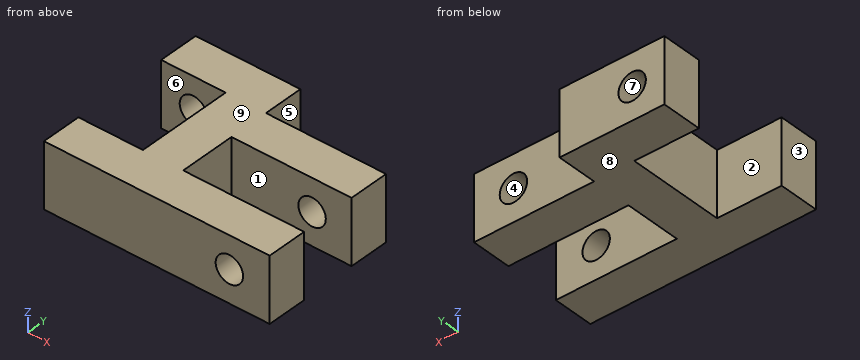
Autodesk Inventor part; units mm, degrees
ref_plane "YZ Plane" through (0, 0, 0) normal (1, 0, 0) x (0, 1, 0)
ref_plane "XZ Plane" through (0, 0, 0) normal (0, 1, 0) x (-1, 0, 0)
ref_plane "XY Plane" through (0, 0, 0) normal (0, 0, 1) x (1, 0, 0)
sketch "Sketch1" plane through (0, 0, 0) normal (0, 0, 1) x (1, 0, 0)
  line L0 (0, 0) -> (15, 0)
  line L1 (15, 0) -> (15, -5)
  line L2 (15, -5) -> (-13, -5)
  line L3 (-13, -5) -> (-13, 0)
  line L4 (-13, 0) -> (-5, 0)
  line L5 (-5, 0) -> (-5, 12)
  line L6 (-5, 12) -> (-13, 12)
  line L7 (-13, 12) -> (-13, 17)
  line L8 (14.8978, 12) -> (14.8978, 7)
  line L9 (14.8978, 7) -> (0, 7)
  line L10 (0, 7) -> (0, 0)
  line L11 (-13, 17) -> (0, 17)
  line L12 (0, 17) -> (0, 12)
  line L13 (0, 12) -> (14.8978, 12)
  dimension "d0" = 15
  dimension "d1" = 5
  dimension "d2" = 28
  dimension "d3" = 5
  dimension "d4" = 8
  dimension "d5" = 12
  dimension "d6" = 8
  dimension "d7" = 5
  dimension "d9" = 5
  dimension "d19" = 5
extrude "Extrusion1" add sketch "Sketch1" along normal blind 8
sketch "Sketch3" plane through (-13, 17, 0) normal (0, 1, 0) x (1, 0, 0)
  line L0 (0, 0) -> (0, -8)
  line L1 (13, 0) -> (13, -8)
  circle A0 centre (23, -4) radius 1.7
  circle A1 centre (4, -4) radius 1.7
  point P0 (13, -4)
  point P1 (13, -4)
  dimension "d20" = 3.4
  dimension "d21" = 3.4
  dimension "d22" = 4
  dimension "d23" = 10
extrude "Extrusion3" cut sketch "Sketch3" against normal blind 30
delete faces "Delete Face1" heal yes whole lump no faces at (-7.322, -3.3333, 4.2727)
properties part number "Pulley vice"
Here's how the part is built. I have some questions about the finished solid (model axes, mm). Face numbers are marked on the shaded views. A direction names the side the tool comes from. Coordinates: 2 decimals unless noted, no trailing zeros. Order: outer loops, then holes, each group sorted by start corner. A loop starts at its lowest first (then second) coordinate and runs counter-clockwise, first axis right, second up. Notation, with made-up numbers: M 2.5,35 L 35.5,35 A16 ccw 35.5,45 Z; hole C 52,62 d4. An arc over 180 degrees is marked long. Answer as a JSON object with one key per item and string values. Group by question number.
(1) For pin 1 (2.5 mm diameter, centred on y = 15, z = 4.5, fed in from +X); pin 2 (3 mm diameter, centred on x = -9, z = 4, fed in from +Y); pin 3 (1.5 mm diameter, centred on y = 8.5, z = 4.5, fed in from +X), each with a flat end and sliding along its axis, tell me the tip position at first contact or that it passes through.
(2) If we mould it in two halves opening along Z, with no side actions, what happens to the marked faces 6, 7, 8 and 9? For each: released by +Z, released by -Z, zero draft, split by the parting line, or undercut.
(3) Suppose I cut it at D-D, the plane y = 15.25. Please give me the cut outline in (x, z).
(4) Suppose I cut it at C-C, the plane x = -9. Please give me the cut outline in (y, z), then the cut area to 3 significant figures.
(5) Which directions (+Z, -Z, +X, -X, +Y, -Y) give clear straight access to the entire face, cutting with the end or side of a thin tool? Please do the marked faces 1, 2, 3, 4 and 5.
(6) I need wall thicknesses on probe 1 along X at (y, z) = (13.45, 4); probe 2 along X at (y, z) = (-2.7, 4); probe 3 along Z at (x, y) = (-9, 13.1). Which ranges of each line are inside material? Lowest first, please.
(7) Suppose I cut it at B-B, the plane x = 7.25. Please give me the cut outline in (y, z).
(8) Suppose I cut it at A-A, the plane z = 4. Please give me the cut outline in (x, y), then the cut area to 3 significant figures.
Values found:
{
 "1": {"pin 1": "stops at x = 0", "pin 2": "stops at y = 0", "pin 3": "stops at x = 14.9"},
 "2": {"face 6": "zero draft", "face 7": "undercut", "face 8": "released by -Z", "face 9": "released by +Z"},
 "3": {"outline": "M -13,0 L 0,0 L 0,8 L -13,8 Z; hole C -9,4 d3.4"},
 "4": {"outline": "M -5,0 L 0,0 L 0,8 L -5,8 Z; M 12,0 L 17,0 L 17,2.3 L 12,2.3 Z; M 12,5.7 L 17,5.7 L 17,8 L 12,8 Z", "area": "63.0 mm^2"},
 "5": {"face 1": "+Z, -Z, +X", "face 2": "+Z, -Z, -X", "face 3": "+Z, -Z, -X, +Y, -Y", "face 4": "+Y, -Y", "face 5": "+Z, -Z, +X, +Y"},
 "6": {"probe 1": "x = -13 to -10.7, -7.3 to 0", "probe 2": "x = -13 to 8.3, 11.7 to 15", "probe 3": "z = 0 to 2.3, 5.7 to 8"},
 "7": {"outline": "M -5,0 L 0,0 L 0,8 L -5,8 Z; M 7,0 L 12,0 L 12,8 L 7,8 Z"},
 "8": {"outline": "M -13,-5 L 8.3,-5 L 8.3,0 L 0,0 L 0,7 L 8.3,7 L 8.3,12 L 0,12 L 0,17 L -7.3,17 L -7.3,12 L -5,12 L -5,0 L -13,0 Z; M -13,12 L -10.7,12 L -10.7,17 L -13,17 Z; M 11.7,-5 L 15,-5 L 15,0 L 11.7,0 Z; M 11.7,7 L 14.9,7 L 14.9,12 L 11.7,12 Z", "area": "288 mm^2"}
}
